The listing builds one solid part. Answer for the finished solid, in the listing's coordinates (mm). A direction names the side the tool comes from. Round coordinates to 2 decimals unless told otherwise and drop trailing zeros. Write each loop counter-clockwise with the first axis right and the second up, starting at its lowest first coordinate (ties: lowest second). Pieces come first, ordered by that corner, then holes. Notation, with made-up numbers: M 82.25,47.5 L 103.25,47.5 A13 ccw 103.25,69.5 Z; hole C -31.5,54 d4. An arc over 180 degrees is marked long. One line per item, written item: value. Start each with the question number.
(1) For a pull along X with two mould halves and no side action, classify faces 5 (the cylindrical face through (-9.788, 24.457, 1.614)), 6 (the flat face through (-8, 0, 9)), 7 (the cylindrical face through (-6.53, 26.08, -5.39)) as released by +X, released by -X, zero draft, split by the parting line, or undercut.
(2) Section D-D (x = -12.25) is taken. Determine the outline of the cut face in (y, z), plus the area to 3 significant figures.
(3) Given P1, Ø0.8, axis at x = -5, z = 9.5, coming from the +Y side; P2, Ø4.5, axis at x = -11.5, z = 0.5, coming from the -Y side; P3, Ø6, axis at y = 8.5, z = -4.5, coming from the +X side, each flat-ended and moving along its own axis, determine where each tip first touches the part or whether it passes through.
(4) Section B-B (x = -6.5) is taken. Determine the outline of the cut face in (y, z), plus the area to 3 significant figures.
(5) For faces 1 (the flat face through (-8, 15.1, 3)), 2 (the flat face through (-9, 25, 3.135)), 3 (the flat face through (-7, 25, -3.865)), 4 (the flat face through (-8.235, -1.726, -5.09)), determine the directions among +Z, -Z, +X, -X, +Y, -Y from which every point of the face is accessible in a straight line to the end or side of a thin tool.
(6) Section A-A (y = 11) is taken. Determine the outline of the cut face in (x, z).
(7) Consider probe 1 along Z at (x, y) = (-1.75, 1.5); probe 2 along Z at (x, y) = (-12, 25); probe 3 along Y at (x, z) = (-5.5, 2). Determine where each line is inside the solid, lowest interval first.
(8) Section C-C (z = 9.5) is taken. Determine the outline of the cut face in (x, y).
```python
from build123d import *

# Parameters (mm, degrees)
SKETCH_1_W        = 15
SKETCH_1_H        = 2
EXTRUDE_1_DEPTH   = 15.1
EXTRUDE_1_2_DEPTH = 15.1
SKETCH_2_W        = 15
SKETCH_2_H        = 19.05
EXTRUDE_2_DEPTH   = 2
EXTRUDE_3_DEPTH   = 15
EXTRUDE_4_DEPTH   = 3
EXTRUDE_5_DEPTH   = 3


with BuildPart() as part:
    # Sketch 1 → Extrude 1 (new body)
    with BuildSketch(Plane(origin=(0, 0, 0), x_dir=(1, 0, 0), z_dir=(0, 1, 0))):
        with Locations((-8.12962963, 5.864814815)):
            Rectangle(SKETCH_1_W, SKETCH_1_H)
    extrude(amount=EXTRUDE_1_DEPTH)



with BuildPart() as body_2:
    # Sketch 1 → Extrude 1 2 (new body)
    with BuildSketch(Plane(origin=(0, 0, 0), x_dir=(1, 0, 0), z_dir=(0, 1, 0))):
        with Locations((-8.12962963, -11.185185185)):
            Rectangle(SKETCH_1_W, SKETCH_1_H)
    extrude(amount=EXTRUDE_1_2_DEPTH)


with BuildPart() as part_1:
    add(part.part)

    add(body_2.part)  # Extrude 2 merges body 2
    # Sketch 2 → Extrude 2 (add)
    with BuildSketch(Plane(origin=(0, 15.1, 0), x_dir=(1, 0, 0), z_dir=(0, 1, 0))):
        with Locations((-8.12962963, -2.660185185)):
            Rectangle(SKETCH_2_W, SKETCH_2_H)
    extrude(amount=EXTRUDE_2_DEPTH)

    # Sketch 3 → Extrude 3 (add)
    with BuildSketch(Plane.ZY.offset(15.62962963)):
        Polygon((-6.864814815, 0), (-3.364814815, 0), (-6.864814815, -3.5), align=None)
        Polygon((12.185185185, 0), (8.685185185, 0), (12.185185185, -3.5), align=None)
    extrude(amount=-EXTRUDE_3_DEPTH)

    # Sketch 5 → Extrude 4 (add)
    with BuildSketch(Plane(origin=(0, 0, -6.864814815), x_dir=(-1, 0, 0), z_dir=(0, 0, -1))):
        with BuildLine():
            Line((14.570760421, 19.888226158), (15.122171723, 19.998508419))
            ThreePointArc((15.122171723, 19.998508419), (15.449589497, 20.226176769), (15.506344599, 20.62090976))
            ThreePointArc((15.506344599, 20.62090976), (6.36809587, 26.042916016), (0.62962963, 17.1))
            Line((0.62962963, 17.1), (2.22962963, 17.1))
            ThreePointArc((2.22962963, 17.1), (6.557748265, 24.481257432), (13.991268777, 20.243528676))
            ThreePointArc((13.991268777, 20.243528676), (14.211351698, 19.952258552), (14.570760421, 19.888226158))
        make_face()
    extrude(amount=-EXTRUDE_4_DEPTH)

    # Sketch 7 → Extrude 5 (add)
    with BuildSketch(Plane.XY.offset(0.135185185)):
        with BuildLine():
            Line((-1.780026825, 19.869920561), (-1.032692548, 20.019387416))
            ThreePointArc((-1.032692548, 20.019387416), (-0.772321289, 20.199010756), (-0.723833364, 20.511591398))
            ThreePointArc((-0.723833364, 20.511591398), (-9.836075513, 26.055738893), (-15.62962963, 17.1))
            Line((-15.62962963, 17.1), (-14.02962963, 17.1))
            ThreePointArc((-14.02962963, 17.1), (-9.659485473, 24.492329005), (-2.245122699, 20.15967246))
            ThreePointArc((-2.245122699, 20.15967246), (-2.069982872, 19.922647762), (-1.780026825, 19.869920561))
        make_face()
    extrude(amount=EXTRUDE_5_DEPTH)


solid = part_1.part
```
Recorded:
1. face 5: undercut
1. face 6: zero draft
1. face 7: split by the parting line
2. outline: M -3.5,-6.86 L 17.1,-6.86 L 17.1,12.19 L -3.5,12.19 L 0,8.69 L 0,10.19 L 15.1,10.19 L 15.1,-4.86 L 0,-4.86 L 0,-3.36 Z; M 23.08,-6.86 L 25.04,-6.86 L 25.04,-3.86 L 23.08,-3.86 Z; M 23.08,0.14 L 25.04,0.14 L 25.04,3.14 L 23.08,3.14 Z
2. area: 123 mm2
3. P1: stops at y = 17.1
3. P2: stops at y = 15.1
3. P3: stops at x = -0.63
4. outline: M -3.5,-6.86 L 17.1,-6.86 L 17.1,12.19 L -3.5,12.19 L 0,8.69 L 0,10.19 L 15.1,10.19 L 15.1,-4.86 L 0,-4.86 L 0,-3.36 Z; M 24.47,-6.86 L 26.07,-6.86 L 26.07,-3.86 L 24.47,-3.86 Z; M 24.47,0.14 L 26.07,0.14 L 26.07,3.14 L 24.47,3.14 Z
4. area: 120 mm2
5. face 1: +X, -X
5. face 2: +Z, +X, -X, +Y
5. face 3: +X, -X, +Y
5. face 4: +X, -X, -Y
6. outline: M -15.63,-6.86 L -0.63,-6.86 L -0.63,-4.86 L -15.63,-4.86 Z; M -15.63,10.19 L -0.63,10.19 L -0.63,12.19 L -15.63,12.19 Z
7. probe 1: z = -6.86 to -4.86, 10.19 to 12.19
7. probe 2: z = -6.86 to -3.86, 0.14 to 3.14
7. probe 3: y = 15.1 to 17.1, 24.09 to 25.78
8. outline: M -15.63,-0.81 L -0.63,-0.81 L -0.63,0 L -15.63,0 Z; M -15.63,15.1 L -0.63,15.1 L -0.63,17.1 L -15.63,17.1 Z
